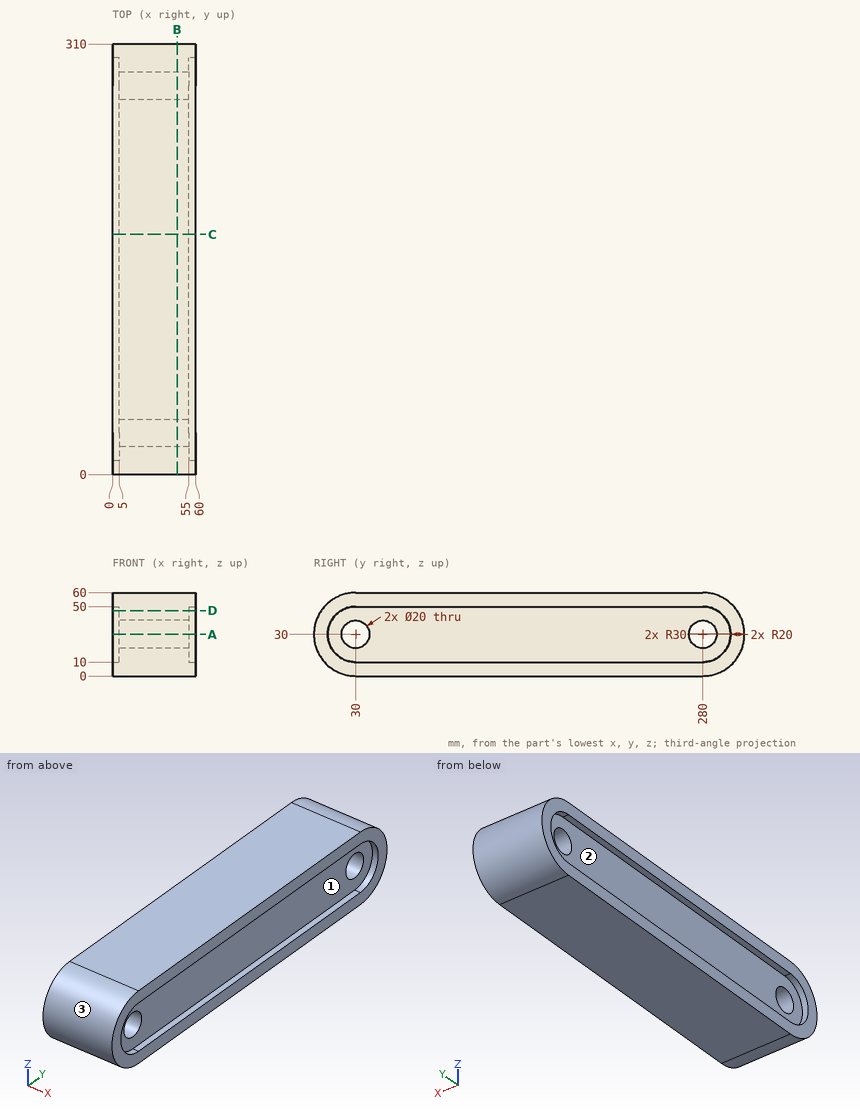
Print and shaded views of the part. All mm, measured from the part's lowest x, y and z. A direction names the side the tool comes from. Coordinates: 2 decimals unless noted, no trailing zeros. Loops run counter-clockwise (first coordinate to the right, second up) from the corner with the lowest first, then second, coordinate; pieces in that order, holes last. Notation, with made-up numbers: (53.25, 30) -> (64.25, 30) arc R9 ccw to (64.25, 43) -> close; hole circle Ø2 at (25.25, 55). An arc over 180 degrees is marked (long way). Use a Markdown table: item, result. Add a question column.
Item 1: Which spindle directions (+Z, -Z, +X, -X, +Y, -Y) get a long thin tool onto all of the face, cutting with end or side? Do the marked faces 1, 2 and 3. Say none if no direction does.
Item 2: Band-saw the part on A-A on z = 30. Write the cut outline in (x, y).
Item 3: Band-saw the part on B-B on x = 46.5. Write the cut outline in (y, z), plus the area to 3 significant figures.
Item 4: Band-saw the part on D-D on z = 47. Write the cut outline in (x, y).
Item 5: Band-saw the part on C-C on y = 173. Write the cut outline in (x, z).
Item 6: Probe probe 1 along Z at (x, y) = (27, 30); probe 2 along Y at (x, z) = (54.5, 31); probe 3 along Z at (x, y) = (57, 58). List the from-to ranges inside material, lowest first.
Item 7: Flat gauge pins, fed straight in: P1, Ø20, axis at y = 104, z = 34.5, coming from the +X side; P2, Ø2, axis at x = 40, z = 42, coming from the +Y side; P3, Ø5, axis at y = 113, z = 20, coming from the -X side. Where does each tip first touch, or does it go through?
Geometry says:
| question | item | result |
|---|---|---|
| 1 | face 1 | +X |
| 1 | face 2 | -X |
| 1 | face 3 | +X, -X, -Y |
| 2 | outline | (0, 0) -> (60, 0) -> (60, 10) -> (55, 10) -> (55, 20) -> (5, 20) -> (5, 10) -> (0, 10) -> close; (0, 300) -> (5, 300) -> (5, 290) -> (55, 290) -> (55, 300) -> (60, 300) -> (60, 310) -> (0, 310) -> close; (5, 40) -> (55, 40) -> (55, 270) -> (5, 270) -> close |
| 3 | outline | (30, 0) -> (280, 0) arc R30 ccw to (280, 60) -> (30, 60) arc R30 ccw to start; hole circle Ø20 at (30, 30); hole circle Ø20 at (280, 30) |
| 3 | area | 17,200 mm² |
| 4 | outline | (0, 5.28) -> (60, 5.28) -> (60, 19.46) -> (55, 19.46) -> (55, 290.54) -> (60, 290.54) -> (60, 304.72) -> (0, 304.72) -> (0, 290.54) -> (5, 290.54) -> (5, 19.46) -> (0, 19.46) -> close |
| 5 | outline | (0, 0) -> (60, 0) -> (60, 10) -> (55, 10) -> (55, 50) -> (60, 50) -> (60, 60) -> (0, 60) -> (0, 50) -> (5, 50) -> (5, 10) -> (0, 10) -> close |
| 6 | probe 1 | 0 to 20, 40 to 60 |
| 6 | probe 2 | 0.02 to 20.05, 39.95 to 270.05, 289.95 to 309.98 |
| 6 | probe 3 | 0 to 10, 50 to 60 |
| 7 | P1 | x = 55 |
| 7 | P2 | y = 307.91 |
| 7 | P3 | x = 5 |
